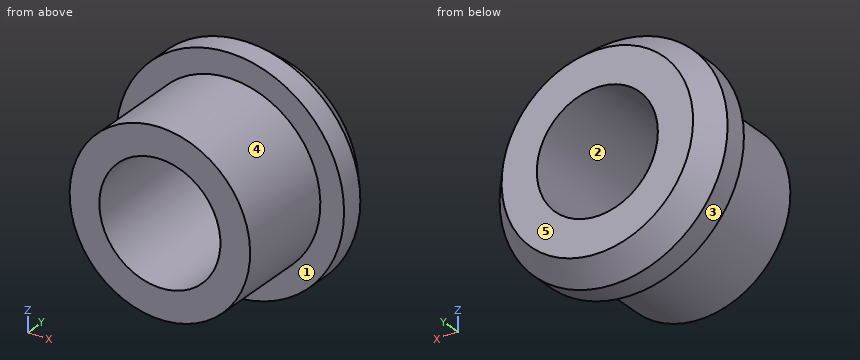
from build123d import *

# Parameters (mm, degrees)
F_3_8_24_TAPPED_HOLE1_D = 8.4328


with BuildPart() as part:
    # Sketch1 → Revolve1 (revolve)
    with BuildSketch(Plane.XY, mode=Mode.PRIVATE) as revolve1_sk:
        Polygon((0, 5.498310654), (0, -4.915689346), (6.2865, -4.915689346), (6.2865, 2.196310654), (7.9375, 2.196310654), (7.9375, 3.847310654), (6.6675, 5.498310654), align=None)
    revolve(revolve1_sk.sketch.rotate(Axis((0, 5.498310654, 0), (0, -1, 0)), 90), axis=Axis((0, 5.498310654, 0), (0, -1, 0)))

    # 3/8-24 Tapped Hole1 (through all)
    with Locations(Plane(origin=(0, 5.498310654, 0), x_dir=(1, 0, 0), z_dir=(0, 1, 0))):
        with Locations((0, 0)):
            Hole(F_3_8_24_TAPPED_HOLE1_D / 2)


solid = part.part
Input: part model. Units: mm. Frame: model coordinates. Face numbers are marked on the shaded views. A direction names the side the tool comes from. Give positions to 0.01 mm unless a question says otherwise; leave off trailing zeros. Loops run counter-clockwise (first coordinate to the right, second up) from the corner with the lowest first, then second, coordinate; pieces in that order, holes last. Notation, with made-up numbers: M 42.25,-23 L 85.25,-23 A25 ccw 85.25,4 Z; hole C 26.5,10 d8. An arc over 180 degrees is marked long. Use CSV: the item, a comma, the result in double quotes.
(1) Section B-B, the plane z = 0. Return loops of the section in (x, y).
Outcome:
outline,"M -7.94,2.2 L -6.29,2.2 L -6.29,-4.92 L -4.22,-4.92 L -4.22,5.5 L -6.67,5.5 L -7.94,3.85 Z; M 4.22,-4.92 L 6.29,-4.92 L 6.29,2.2 L 7.94,2.2 L 7.94,3.85 L 6.67,5.5 L 4.22,5.5 Z"
(2) Pin query (flat end, axial travel): P1, Ø3, axis at y = 1, z = -6, coming from the +X side; P2, Ø3, axis at y = 4, z = -3, coming from the -X side; P3, Ø5, axis at x = -3, y = 2.5, coming from the -Z side. Return the tip coordinate at first contact, or that it passes through.
Outcome:
P1,"stops at x = 6.09"
P2,"stops at x = -7.79"
P3,"stops at z = -7.92"
(3) Section C-C, the plane y = -2.5. Return loops of the section in (x, z), plus the area to 3 significant figures.
Outcome:
outline,"C 0,0 d12.57; hole C 0,0 d8.43"
area,"68.3 mm²"
(4) Set-up query: the marked faces 4 and 5. Return all of +Z, -Z, +X, -X, +Y, -Y with unobstructed straight access to the full face (end or side cutting, diameter ignored); none if empty.
Outcome:
face 4,"-Y"
face 5,"+Z, -Z, +X, -X, +Y"
(5) Section D-D, the plane y = 3. Return loops of the section in (x, z) (1 decimal).
Outcome:
outline,"C 0,0 d15.9; hole C 0,0 d8.4"
(6) Material intervals for L1, parallel to Z at x = -2, y = -1.5; L2, parallel to X at y = -3, z = -1.25, sorted ascending. Write a range as [from, to].
Outcome:
L1,"z = [-5.96, -3.71], [3.71, 5.96]"
L2,"x = [-6.16, -4.03], [4.03, 6.16]"
(7) Section A-A, the plane x = 0. Return loops of the section in (y, z), plus the area to 3 significant figures.
Outcome:
outline,"M -4.92,-6.29 L 2.2,-6.29 L 2.2,-7.94 L 3.85,-7.94 L 5.5,-6.67 L 5.5,-4.22 L -4.92,-4.22 Z; M -4.92,4.22 L 5.5,4.22 L 5.5,6.67 L 3.85,7.94 L 2.2,7.94 L 2.2,6.29 L -4.92,6.29 Z"
area,"51.9 mm²"
(8) Pull-direction query (X, two-part tool) for the marked faces 1, 2 and 3; classes: pulls with the +X half, pulls with the -X half, needs draft (parallel to the pull), parting line crosses it, or undercut.
Outcome:
face 1,"needs draft"
face 2,"undercut"
face 3,"parting line crosses it"
